Read the model definition and answer for the solid it produces. Units are mm, in the model's axes. A direction names the side the tool comes from. Round coordinates to 2 decimals unless told otherwise and drop trailing zeros. Write each loop counter-clockwise with the first axis right and the second up, starting at its lowest first coordinate (ties: lowest second). Pieces come first, ordered by that corner, then holes. Notation, with made-up numbers: (-8.5, 12.5) - (36.5, 12.5) arc R12 ccw to (36.5, 16.5) - close; hole circle Ø8 at (45.5, 32). An arc over 180 degrees is marked (long way). One line per item, written item: value. Start each with the question number.
(1) Find the intervals of material crossed by L1, parallel to X at y = -39, z = 0.5 (3 decimals); L2, parallel to Y at x = -26.5, z = 3 (3 decimals); L3, parallel to X at y = -2.5, z = 1.95 (3 decimals), in increasing order.
(2) A cutting plane is placed at A-A, the plane x = -27.5. Determine the outline of the cut face in (y, z) (3 decimals).
(3) Flat-ended cylindrical pins translate along their axes: pin 1 Ø1 at (y, z) = (-45, 1) entering from +X; pin 2 Ø1.6 at (x, z) = (-77.5, 2) entering from +Y; pin 3 Ø1.6 at (y, z) = (23, 1) entering from -X. Find the tip coordinate at first contact, or state that the pin passes through.
(4) A cutting plane is placed at C-C, the plane y = -6. Determine the outline of the cut face in (x, z) (3 decimals).
(5) The mould has two halves that part along Y. Classify faces 1 (the face through (58, -11, 3.175)), 2 (the face through (20.704, -61.979, 1.565)), 3 (the face through (-20.571, -61.846, 1.565)): +Y half, -Y half, draft (parallel to the pull), parting line (faces both ways), or undercut.
(6) For faces 4 (the face through (58, -11, 0)), 5 (the face through (20.571, 61.846, 1.565)), determine the directions among +Z, -Z, +X, -X, +Y, -Y from which every point of the face is accessible in a straight line to the end or side of a thin tool.
(7) A cutting plane is placed at B-B, the plane z = 1.45. Determine the outline of the cut face in (x, y) (3 decimals), plus the area to 3 significant figures.
from build123d import *

# Parameters (mm, degrees)
SKETCH1_W           = 152.4
SKETCH1_H           = 152.4
SKETCH1_W_2         = 133.35
SKETCH1_H_2         = 133.35
BOSS_EXTRUDE1_DEPTH = 3.175
SKETCH2_W           = 3.175
SKETCH2_H           = 152.4
BOSS_EXTRUDE4_DEPTH = 3.175
SKETCH3_W           = 3.175
SKETCH3_H           = 76.2
BOSS_EXTRUDE5_DEPTH = 3.175
SKETCH4_W           = 3.175
SKETCH4_H           = 76.2
CUT_EXTRUDE1_DEPTH  = 3.175


with BuildPart() as part:
    # Sketch1 → Boss-Extrude1 (new body)
    with BuildSketch(Plane.XY):
        Rectangle(SKETCH1_W, SKETCH1_H)
        Rectangle(SKETCH1_W_2, SKETCH1_H_2, mode=Mode.SUBTRACT)
        Polygon((25.4, 66.675), (-25.4, 66.675), (-15.875, 57.15), (15.875, 57.15), align=None)
        Polygon((66.675, -25.4), (66.675, 25.4), (57.15, 15.875), (57.15, -15.875), align=None)
        Polygon((-15.875, -57.15), (-25.4, -66.675), (25.4, -66.675), (15.875, -57.15), align=None)
        Polygon((-57.15, 15.875), (-66.675, 25.4), (-66.675, -25.4), (-57.15, -15.875), align=None)
    extrude(amount=BOSS_EXTRUDE1_DEPTH)

    # Sketch2 → Boss-Extrude4 (add)
    with BuildSketch(Plane.XY.offset(3.175)):
        with Locations((77.7875, 0)):
            Rectangle(SKETCH2_W, SKETCH2_H)
    extrude(amount=-BOSS_EXTRUDE4_DEPTH)

    # Sketch3 → Boss-Extrude5 (add)
    with BuildSketch(Plane.XY.offset(3.175)):
        with Locations((77.7875, 38.1)):
            Rectangle(SKETCH3_W, SKETCH3_H)
        with Locations((-77.7875, -38.1)):
            Rectangle(SKETCH3_W, SKETCH3_H)
    extrude(amount=-BOSS_EXTRUDE5_DEPTH)

    # Sketch4 → Cut-Extrude1 (cut)
    with BuildSketch(Plane.XY.offset(3.175)):
        with Locations((77.7875, -38.1)):
            Rectangle(SKETCH4_W, SKETCH4_H)
    extrude(amount=-CUT_EXTRUDE1_DEPTH, mode=Mode.SUBTRACT)


solid = part.part
Here are the results:
1. L1: -79.375 to -66.675, 66.675 to 76.2
1. L2: -76.2 to -66.675, 66.675 to 76.2
1. L3: -79.375 to -57.15, 57.15 to 76.2
2. outline: (-76.2, 0) - (-66.675, 0) - (-66.675, 3.175) - (-76.2, 3.175) - close; (66.675, 0) - (76.2, 0) - (76.2, 3.175) - (66.675, 3.175) - close
3. pin 1: x = 76.2
3. pin 2: y = 0
3. pin 3: x = -76.2
4. outline: (-79.375, 0) - (-57.15, 0) - (-57.15, 3.175) - (-79.375, 3.175) - close; (57.15, 0) - (76.2, 0) - (76.2, 3.175) - (57.15, 3.175) - close
5. face 1: draft
5. face 2: undercut
5. face 3: undercut
6. face 4: -Z, +X, -X, +Y, -Y
6. face 5: +Z, -Z
7. outline: (-79.375, -76.2) - (76.2, -76.2) - (76.2, 0) - (79.375, 0) - (79.375, 76.2) - (-76.2, 76.2) - (-76.2, 0) - (-79.375, 0) - close; hole (-66.675, -66.675) - (-25.4, -66.675) - (-15.875, -57.15) - (15.875, -57.15) - (25.4, -66.675) - (66.675, -66.675) - (66.675, -25.4) - (57.15, -15.875) - (57.15, 15.875) - (66.675, 25.4) - (66.675, 66.675) - (25.4, 66.675) - (15.875, 57.15) - (-15.875, 57.15) - (-25.4, 66.675) - (-66.675, 66.675) - (-66.675, 25.4) - (-57.15, 15.875) - (-57.15, -15.875) - (-66.675, -25.4) - close
7. area: 7,500 mm²
